```python
from build123d import *

# Parameters (mm, degrees)
F0_W        = 3
F0_H        = 2.5
F0_H_2      = 39
F1_DEPTH    = 2
F0_W_2      = 3.5
F0_W_3      = 29.5
F0_R        = 6.5
F2_DEPTH    = 4
F3_T1_DEPTH = 13.9242400177
F3_T3_DEPTH = 14.5
F3_T5_DEPTH = 27


# Not quite as in the source:
# - a fillet or chamfer that OpenCascade refuses, or shapes differently, is made with other operations: its cross-section is extruded or revolved along the edge and cut away or added


with BuildPart() as f1:
    # F0 (on Top) → F1 (new body)
    with BuildSketch(Plane.XY):
        Polygon((20.5, -22), (20.5, 22), (-11.5, 22), (-11.5, 19.5), (18, 19.5), (18, -19.5), (-11.5, -19.5), (-11.5, -22), align=None)
        with Locations((-13, 20.75)):
            Rectangle(F0_W, F0_H)
        Polygon((-14.5, 19.5), (-14.5, 22), (-20.5, 22), (-20.5, -22), (-14.5, -22), (-14.5, -19.5), (-18, -19.5), (-18, 19.5), align=None)
        with Locations((-13, -20.75)):
            Rectangle(F0_W, F0_H)
        with Locations((-13, 0)):
            Rectangle(F0_W, F0_H_2)
    extrude(amount=F1_DEPTH)

    # F0 (on Top) → F2 (join)
    with BuildSketch(Plane.XY):
        with Locations((-16.25, 0)):
            Rectangle(F0_W_2, F0_H_2)
        with Locations((3.25, 0)):
            Rectangle(F0_W_3, F0_H_2)
        with Locations((5, 0.5)):
            Circle(F0_R, mode=Mode.SUBTRACT)
    extrude(amount=F2_DEPTH)

    # F3: fillet of radius 5 on 8 edges, made by hand

    # F3_s2 → F3_t1 (cut)
    with BuildSketch(Plane.XY.offset(2)):
        with BuildLine():
            ThreePointArc((-18, 14.7303039929), (-17.0311288741, 17.6883438845), (-14.5, 19.5))
            Line((-14.5, 19.5), (-18, 19.5))
            Line((-18, 19.5), (-18, 14.7303039929))
        make_face()
        with BuildLine():
            ThreePointArc((-18, -14.7303039929), (-17.0311288741, -17.6883438845), (-14.5, -19.5))
            Line((-14.5, -19.5), (-18, -19.5))
            Line((-18, -19.5), (-18, -14.7303039929))
        make_face()
    extrude(amount=F3_T1_DEPTH, mode=Mode.SUBTRACT)

    # F3_s4 → F3_t3 (cut)
    with BuildSketch(Plane.XY.offset(2)):
        with BuildLine():
            ThreePointArc((13, 19.5), (16.5355339059, 18.0355339059), (18, 14.5))
            Line((18, 14.5), (18, 19.5))
            Line((18, 19.5), (13, 19.5))
        make_face()
        with BuildLine():
            ThreePointArc((18, -14.5), (16.5355339059, -18.0355339059), (13, -19.5))
            Line((13, -19.5), (18, -19.5))
            Line((18, -19.5), (18, -14.5))
        make_face()
    extrude(amount=F3_T3_DEPTH, mode=Mode.SUBTRACT)

    # F3_s6 → F3_t5 (cut)
    with BuildSketch(Plane.XY.offset(-12.5)):
        with BuildLine():
            ThreePointArc((-15.5, 22), (-19.0355339059, 20.5355339059), (-20.5, 17))
            Line((-20.5, 17), (-20.5, 22))
            Line((-20.5, 22), (-15.5, 22))
        make_face()
        with BuildLine():
            ThreePointArc((-15.5, -22), (-19.0355339059, -20.5355339059), (-20.5, -17))
            Line((-20.5, -17), (-20.5, -22))
            Line((-20.5, -22), (-15.5, -22))
        make_face()
        with BuildLine():
            ThreePointArc((20.5, 17), (19.0355339059, 20.5355339059), (15.5, 22))
            Line((15.5, 22), (20.5, 22))
            Line((20.5, 22), (20.5, 17))
        make_face()
        with BuildLine():
            ThreePointArc((20.5, -17), (19.0355339059, -20.5355339059), (15.5, -22))
            Line((15.5, -22), (20.5, -22))
            Line((20.5, -22), (20.5, -17))
        make_face()
    extrude(amount=F3_T5_DEPTH, mode=Mode.SUBTRACT)


solid = f1.part
```
Geometry: final body of the model. Coordinates: model frame, mm. A direction names the side the tool comes from. Round coordinates to 2 decimals unless told otherwise and drop trailing zeros. Write each loop counter-clockwise with the first axis right and the second up, starting at its lowest first coordinate (ties: lowest second). Pieces come first, ordered by that corner, then holes.
Item 1: Mould query, pull axis Y, two halves, no side actions, for faces 1 (the face through (-12, 2, 2)), 2 (the face through (19.07, 20.5, 0.99)), 3 (the face through (-19, -20.57, 0.99)), 4 (the face through (11.2, 2.45, 1.97)). Classes: +Y half, -Y half, draft (parallel to the pull), parting line (faces both ways), or undercut.
Item 2: Section query B-B (y = -5.5). Return loops of the section in (x, z), plus the area to 3 significant figures.
Item 3: Material intervals for L1, parallel to Y at x = 5, z = 1.2; L2, parallel to X at y = -1, z = 3.8; L3, parallel to X at y = -7.5, z = 2.4, sorted ascending.
Item 4: Section query C-C (x = 5). Return loops of the section in (y, z), plus the area to 3 significant figures.
Item 5: Section query D-D (y = 0.5). Return loops of the section in (x, z), plus the area to 3 significant figures.
Item 6: Set-up query: faces 5 (the face through (-17.06, -17.65, 2.99)), 6 (the face through (-17.06, 17.65, 2.99)), 7 (the face through (-18, 0, 3)), 8 (the face through (-11.5, 0, 3)), 9 (the face through (16.57, -18, 2.99)). Return all of +Z, -Z, +X, -X, +Y, -Y with unobstructed straight access to the full face (end or side cutting, diameter ignored); none if empty.
Item 7: Pin query (flat end, axial travel): P1, Ø0.6, axis at y = 5.5, z = 3, coming from the +X side; P2, Ø1.6, axis at y = -2.5, z = 2.5, coming from the -X side; P3, Ø1.6, axis at x = 3.5, z = 3.5, coming from the +Y side; P4, Ø0.6, axis at x = 0.5, z = 2.5, coming from the -Y side. Return the tip coordinate at first contact, or that it passes through.
Item 8: Section query A-A (z = 2.65). Return loops of the section in (x, y).
Completed:
1. face 1: draft
1. face 2: +Y half
1. face 3: -Y half
1. face 4: undercut
2. outline: (-20.5, 0) - (2.5, 0) - (2.5, 4) - (-11.5, 4) - (-11.5, 2) - (-14.5, 2) - (-14.5, 4) - (-18, 4) - (-18, 2) - (-20.5, 2) - close; (7.5, 0) - (20.5, 0) - (20.5, 2) - (18, 2) - (18, 4) - (7.5, 4) - close
2. area: 128 mm2
3. L1: y = -22 to -6, 7 to 22
3. L2: x = -18 to -14.5, -11.5 to -1.32, 11.32 to 18
3. L3: x = -18 to -14.5, -11.5 to 18
4. outline: (-22, 0) - (-6, 0) - (-6, 4) - (-19.5, 4) - (-19.5, 2) - (-22, 2) - close; (7, 0) - (22, 0) - (22, 2) - (19.5, 2) - (19.5, 4) - (7, 4) - close
4. area: 114 mm2
5. outline: (-20.5, 0) - (-1.5, 0) - (-1.5, 4) - (-11.5, 4) - (-11.5, 2) - (-14.5, 2) - (-14.5, 4) - (-18, 4) - (-18, 2) - (-20.5, 2) - close; (11.5, 0) - (20.5, 0) - (20.5, 2) - (18, 2) - (18, 4) - (11.5, 4) - close
5. area: 96.0 mm2
6. face 5: +Z, -X, -Y
6. face 6: +Z, -X, +Y
6. face 7: +Z, -X, +Y, -Y
6. face 8: +Z, +Y, -Y
6. face 9: +Z, +X, -Y
7. P1: stops at x = 18
7. P2: stops at x = -20.5
7. P3: stops at y = 19.5
7. P4: stops at y = -19.5
8. outline: (-18, -14.73) arc R5 ccw to (-14.5, -19.5) - (-14.5, 19.5) arc R5 ccw to (-18, 14.73) - close; (-11.5, -19.5) - (13, -19.5) arc R5 ccw to (18, -14.5) - (18, 14.5) arc R5 ccw to (13, 19.5) - (-11.5, 19.5) - close; hole circle Ø13 at (5, 0.5)
